```python
from build123d import *

# Parameters (mm, degrees)
F0_W     = 71.0946
F0_H     = 30.48
F1_DEPTH = 25.4
F2_T     = -2.54
F4_D     = 3.81


with BuildPart() as f1:
    # F0 (on Top) → F1 (new body)
    with BuildSketch(Plane.XY):
        Rectangle(F0_W, F0_H)
    extrude(amount=F1_DEPTH)

    # F2
    f2_openings = [f1.faces().sort_by_distance(p)[0] for p in [
        (0, 15.24, 12.7),
        (0, 0, 25.4),
    ]]
    offset(amount=F2_T, openings=f2_openings)

    # F4 (through all)
    with Locations(Plane.XZ.offset(15.24)):
        with Locations((0, 5.320419)):
            Hole(F4_D / 2)


solid = f1.part
```
The model under review builds one solid part; all positions refer to its coordinate system, in mm. A direction names the side the tool comes from. Round coordinates to 2 decimals unless told otherwise and drop trailing zeros. Order: outer loops, then holes, each group sorted by start corner. A loop starts at its lowest first (then second) coordinate and runs counter-clockwise, first axis right, second up. Notation, with made-up numbers: (14, 69.25) -> (66, 69.25) arc R16 cw to (66, 97.25) -> close; hole circle Ø4 at (68.5, 1.25). An arc over 180 degrees is marked (long way). Use a Markdown table: item, result.
Q1. For line 1 (Z direction, x = 0, y = -13.4); line 2 (X direction, y = 13, z = 5.5); line 3 (Y direction, x = 7.5, z = 16), list the stretches that pass through material, from the lowest coordinate up.
Values:
| item | result |
|---|---|
| line 1 | z = 0 to 3.42, 7.23 to 25.4 |
| line 2 | x = -35.55 to -33.01, 33.01 to 35.55 |
| line 3 | y = -15.24 to -12.7 |
Q2. We need section A-A on x = 0. Write out the cut boundary in (y, z), then the cut area to 3 significant figures.
Values:
| item | result |
|---|---|
| outline | (-15.24, 0) -> (15.24, 0) -> (15.24, 2.54) -> (-12.7, 2.54) -> (-12.7, 3.42) -> (-15.24, 3.42) -> close; (-15.24, 7.23) -> (-12.7, 7.23) -> (-12.7, 25.4) -> (-15.24, 25.4) -> close |
| area | 126 mm^2 |
Q3. We need section D-D on y = 2. Write out the cut boundary in (x, z), then the cut area to 3 significant figures.
Values:
| item | result |
|---|---|
| outline | (-35.55, 0) -> (35.55, 0) -> (35.55, 25.4) -> (33.01, 25.4) -> (33.01, 2.54) -> (-33.01, 2.54) -> (-33.01, 25.4) -> (-35.55, 25.4) -> close |
| area | 297 mm^2 |
Q4. We need section B-B on z = 9.75. Write out the cut boundary in (x, y), then the cut area to 3 significant figures.
Values:
| item | result |
|---|---|
| outline | (-35.55, -15.24) -> (35.55, -15.24) -> (35.55, 15.24) -> (33.01, 15.24) -> (33.01, -12.7) -> (-33.01, -12.7) -> (-33.01, 15.24) -> (-35.55, 15.24) -> close |
| area | 323 mm^2 |
Q5. We need section C-C on x = 17. Write out the cut boundary in (y, z).
Values:
| item | result |
|---|---|
| outline | (-15.24, 0) -> (15.24, 0) -> (15.24, 2.54) -> (-12.7, 2.54) -> (-12.7, 25.4) -> (-15.24, 25.4) -> close |
Q6. Tool access review of faces 4 (the flat face through (-33.007, 1, 14)), 5 (the flat face through (0, -13, 25.4)): name each direction out of +Z, -Z, +X, -X, +Y, -Y from which nothing blocks a thin tool from reaching the whole face with its end or side.
Values:
| item | result |
|---|---|
| face 4 | +Z, +Y |
| face 5 | +Z, +X, -X, +Y, -Y |
Q7. Mouldability with a two-part tool opening along X and no side actions: class faces 1 (the cylindrical face through (0.25, -13.95, 7.21)), 2 (the flat face through (-35.547, 0, 13)), 3 (the flat face through (0, -15.24, 13)) as +X half, -X half, draft (parallel to the pull), parting line (faces both ways), or undercut.
Values:
| item | result |
|---|---|
| face 1 | undercut |
| face 2 | -X half |
| face 3 | draft |
Q8. Clearance check with flat-ended pins moving along their axes: P1, Ø12, axis at x = 20, y = -3.5, coming from the -Z side; P2, Ø8, axis at x = -18, z = 13.5, coming from the +Y side; P3, Ø14, axis at x = -12, y = 3, coming from the +Z side; P4, Ø3.5, axis at x = 0, z = 5.32, coming from the +Y side. State where each tip first meets the part, or that it passes through.
Values:
| item | result |
|---|---|
| P1 | stops at z = 0 |
| P2 | stops at y = -12.7 |
| P3 | stops at z = 2.54 |
| P4 | passes through |
